Autodesk Inventor part; units mm, degrees
ref_plane "Plano de trabajo2" through (33.88, 0, 75) normal (-1, 0, 0) x (0, 0, 1)
ref_plane "YZ Plane" through (0, 0, 0) normal (1, 0, 0) x (0, 1, 0)
ref_plane "XZ Plane" through (0, 0, 0) normal (0, 1, 0) x (-1, 0, 0)
ref_plane "Plano de trabajo2" through (33.88, 0, 75) normal (-1, 0, 0) x (0, 0, 1)
sketch "Boceto2" plane through (0, 0, 0) normal (1, 0, 0) x (0, 1, 0)
  line L0 (0, 0) -> (3, 0)
  line L1 (3, 0) -> (3, 78)
  line L2 (3, 78) -> (0, 78)
  line L3 (0, 78) -> (0, 0)
  dimension "d4" = 3
  dimension "d5" = 78
extrude "Extrusión2" add sketch "Boceto2" along normal up to surface (33.88 mm away)
sketch "Boceto3" plane through (0, 3, 78) normal (0, 1, 0) x (1, 0, 0)
  circle A0 centre (3, 3) radius 2.1
  circle A1 centre (30.88, 3) radius 2.1
  circle A2 centre (3, 75) radius 2.1
  circle A3 centre (28.88, 75) radius 2.1
  point P0 (0, 78)
hole "Agujero1" at (3, 3, 75) at (30.88, 3, 75) at (3, 3, 3) at (28.88, 3, 3) direction (0, -1, 0) diameter 3 depth 5
properties part number "Lateral trasero"
Read the model definition and answer for the solid it produces. Units are mm, in the model's axes. Coordinates: 2 decimals unless noted, no trailing zeros. Loops run counter-clockwise (first coordinate to the right, second up) from the corner with the lowest first, then second, coordinate; pieces in that order, holes last. Notation, with made-up numbers: (89.5, -12.5) - (116.5, -12.5) arc R18 cw to (116.5, 9.5) - close; hole circle Ø8 at (42.25, -5). An arc over 180 degrees is marked (long way). Answer in a Markdown table with one row per item.
1. Straight lines are drawn through the part: line 1 (X direction, y = 1.3, z = 75); line 2 (Z direction, x = 3, y = 1.05); line 3 (X direction, y = 0.9, z = 3). For each, find the intervals that lie inside material, in ascending order.
Conclusion:
| item | result |
|---|---|
| line 1 | x = 0 to 1.5, 4.5 to 29.38, 32.38 to 33.88 |
| line 2 | z = 0 to 1.5, 4.5 to 73.5, 76.5 to 78 |
| line 3 | x = 0 to 1.5, 4.5 to 27.38, 30.38 to 33.88 |
2. Find section B-B, the plane z = 75. Write down the section's boundary in (x, y), then the cut area to 3 significant figures.
Conclusion:
| item | result |
|---|---|
| outline | (0, 0) - (1.5, 0) - (1.5, 3) - (0, 3) - close; (4.5, 0) - (29.38, 0) - (29.38, 3) - (4.5, 3) - close; (32.38, 0) - (33.88, 0) - (33.88, 3) - (32.38, 3) - close |
| area | 83.6 mm² |
3. Determine the mould class of faces 1 (the face through (17, 2, 78)), 2 (the face through (17, 3, 38)), 3 (the face through (31.455, 1.479, 76.386)) for opening direction Z: +Z half, -Z half, draft (parallel to the pull), parting line (faces both ways), or undercut.
Conclusion:
| item | result |
|---|---|
| face 1 | +Z half |
| face 2 | draft |
| face 3 | undercut |
4. Find section A-A, the plane x = 3. Write down the section's boundary in (y, z), then the cut area to 3 significant figures.
Conclusion:
| item | result |
|---|---|
| outline | (0, 0) - (3, 0) - (3, 1.5) - (0, 1.5) - close; (0, 4.5) - (3, 4.5) - (3, 73.5) - (0, 73.5) - close; (0, 76.5) - (3, 76.5) - (3, 78) - (0, 78) - close |
| area | 216 mm² |
